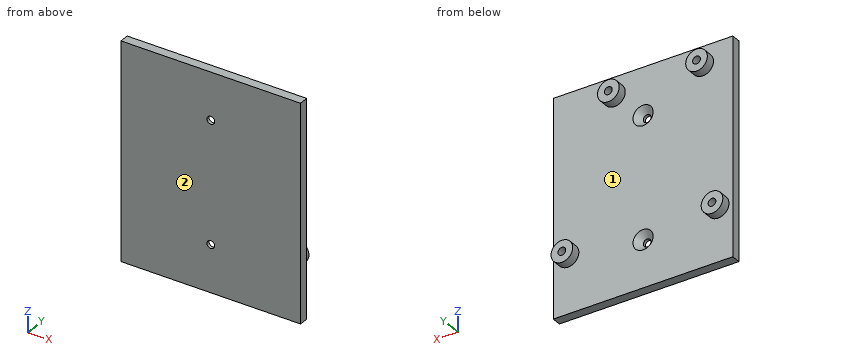
```python
from build123d import *

# Parameters (mm, degrees)
SKETCH_1_W          = 58
SKETCH_1_H          = 70
EXTRUDE_1_DEPTH     = 3
SKETCH_2_R          = 3.5
SKETCH_2_R_2        = 1.25
EXTRUDE_2_DEPTH     = 3
SKETCH_3_R          = 1.25
CUT_EXTRUDE_1_DEPTH = 3
CHAMFER_1_SIZE      = 2


with BuildPart() as part:
    # Эскиз1 → Бобышка-Вытянуть1 (new body)
    with BuildSketch(Plane(origin=(0, 0, 0), x_dir=(1, 0, 0), z_dir=(0, 1, 0))):
        with Locations((4.058065061, -21.04666133)):
            Rectangle(SKETCH_1_W, SKETCH_1_H)
    extrude(amount=EXTRUDE_1_DEPTH)

    # Эскиз2 → Бобышка-Вытянуть2 (add)
    with BuildSketch(Plane(origin=(0, 3, 0), x_dir=(1, 0, 0), z_dir=(0, 1, 0))):
        with Locations((28.308065061, -4.39666133)):
            Circle(SKETCH_2_R)
        with Locations((28.308065061, -4.39666133)):
            Circle(SKETCH_2_R_2, mode=Mode.SUBTRACT)
        with Locations((-20.191934939, -3.39666133)):
            Circle(SKETCH_2_R)
        with Locations((-20.191934939, -3.39666133)):
            Circle(SKETCH_2_R_2, mode=Mode.SUBTRACT)
        with Locations((-15.191934939, -50.19666133)):
            Circle(SKETCH_2_R)
        with Locations((-15.191934939, -50.19666133)):
            Circle(SKETCH_2_R_2, mode=Mode.SUBTRACT)
        with Locations((13.308065061, -50.19666133)):
            Circle(SKETCH_2_R)
        with Locations((13.308065061, -50.19666133)):
            Circle(SKETCH_2_R_2, mode=Mode.SUBTRACT)
    extrude(amount=EXTRUDE_2_DEPTH)

    # Эскиз3 → Вырез-Вытянуть1 (cut)
    with BuildSketch(Plane(origin=(0, 3, 0), x_dir=(1, 0, 0), z_dir=(0, 1, 0))):
        with Locations((4.058065061, -1.335122264)):
            Circle(SKETCH_3_R)
        with Locations((4.058065061, -40.758200397)):
            Circle(SKETCH_3_R)
    extrude(amount=-CUT_EXTRUDE_1_DEPTH, mode=Mode.SUBTRACT)

    # Фаска1
    chamfer_1_edges = [part.edges().sort_by_distance(p)[0] for p in [
        (2.808065061, 3, 1.335122264),
        (2.808065061, 3, 40.758200397),
    ]]
    chamfer(chamfer_1_edges, length=CHAMFER_1_SIZE)


solid = part.part
```
Work out the finished part from the listing and answer in its coordinate system (mm). Face numbers are marked on the shaded views. A direction names the side the tool comes from. Coordinates: 2 decimals unless noted, no trailing zeros. Write each loop counter-clockwise with the first axis right and the second up, starting at its lowest first coordinate (ties: lowest second). Pieces come first, ordered by that corner, then holes. Notation, with made-up numbers: (9.5, 49) - (60.5, 49) arc R31 ccw to (60.5, 76) - close; hole circle Ø7 at (23.5, -31). An arc over 180 degrees is marked (long way). Answer as a JSON object with one key per item and string values.
Q1. Find section D-D (z = 22.5). Write down the section's boundary in (x, y), plus the area to 3 significant figures.
Results list:
{"outline": "(-24.94, 0) - (33.06, 0) - (33.06, 3) - (-24.94, 3) - close", "area": "174 mm^2"}
Q2. Consider L1, parallel to X at y = 0.45, z = 1.5; L2, parallel to Z at x = 5, y = 2.8; L3, parallel to X at y = 3.6, z = 3. Determine where each line is inside the solid, lowest interval first. Write a range as from..to.
Results list:
{"L1": "x = -24.94..2.82, 5.3..33.06", "L2": "z = -13.95..-1.57, 4.24..37.86, 43.66..56.05", "L3": "x = -23.67..-21.38, -19.01..-16.71, 25.1..31.52"}
Q3. Which of the six approach directions +Z, -Z, +X, -X, +Y, -Y give full straight-line access (tool end or side, diameter ignored) to the marked faces 1 and 2?
Results list:
{"face 1": "+Y", "face 2": "+Z, -Z, +X, -X, -Y"}
Q4. Find section B-B (z = 48). Write down the section's boundary in (x, y), plus the area to 3 significant figures.
Results list:
{"outline": "(-24.94, 0) - (33.06, 0) - (33.06, 3) - (16.03, 3) - (16.03, 6) - (10.58, 6) - (10.58, 3) - (-12.47, 3) - (-12.47, 6) - (-17.92, 6) - (-17.92, 3) - (-24.94, 3) - close", "area": "207 mm^2"}
Q5. Given pin 1 Ø3 at (x, z) = (4.06, 1.34) entering from -Y; pin 2 Ø2 at (x, z) = (28.31, 4.4) entering from +Y; pin 3 Ø1.5 at (y, z) = (5.5, -1) entering from +X, each flat-ended and moving along its own axis, determine where each tip first touches the part or whether it passes through.
Results list:
{"pin 1": "stops at y = 0", "pin 2": "stops at y = 3", "pin 3": "passes through"}
Q6. Find section C-C (x = 19.5). Write down the section's boundary in (y, z), plus the area to 3 significant figures.
Results list:
{"outline": "(0, -13.95) - (3, -13.95) - (3, 56.05) - (0, 56.05) - close", "area": "210 mm^2"}
Q7. Find section A-A (y = 5). Write down the section's boundary in (x, z), plus the area to 3 significant figures.
Results list:
{"outline": "circle Ø7 at (-20.19, 3.4); circle Ø7 at (-15.19, 50.2); circle Ø7 at (13.31, 50.2); circle Ø7 at (28.31, 4.4); hole circle Ø2.5 at (-20.19, 3.4); hole circle Ø2.5 at (-15.19, 50.2); hole circle Ø2.5 at (13.31, 50.2); hole circle Ø2.5 at (28.31, 4.4)", "area": "134 mm^2"}
